Part model, mm, in its own coordinate system. A direction names the side the tool comes from. Coordinates: 2 decimals unless noted, no trailing zeros. Loops run counter-clockwise (first coordinate to the right, second up) from the corner with the lowest first, then second, coordinate; pieces in that order, holes last. Notation, with made-up numbers: (43, -4) - (53, -4) arc R38 cw to (53, 35) - close; hole circle Ø7 at (14.5, 87.5). An arc over 180 degrees is marked (long way). Use a Markdown table: item, result. Add a question column.
1. Band-saw the part on A-A, the plane z = 0.6. Give the cut face in (x, y) (3 decimals).
2. Wall check: probe 1 along X at (y, z) = (-5, 2.9); probe 2 along Y at (x, z) = (2.5, 0.95) (3 decimals); probe 3 along Y at (x, z) = (12.5, 0.55) (3 decimals). Give the ranges that are in metal, low to high. Write a range as [from, to].
3. Band-saw the part on B-B, the plane x = 9.5. Give the cut face in (y, z) (3 decimals), plus the area to 3 significant figures.
4. Pull direction X, two halves, no side cores. Call faces 3 (the flat face through (-19.05, 0, 2)), 4 (the flat face through (0, 0, 0)), 5 (the flat face through (0, -11.049, 2)): pulls with the +X half, pulls with the -X half, needs draft (parallel to the pull), parting line crosses it, or undercut.
5. Drop flat-ended pins along their axis: pin 1 (3 mm diameter, centred on x = 7, y = -1, fed in from +Z); pin 2 (10 mm diameter, centred on x = 15, y = 1, fed in from +Z). Give the stop position or say it passes through.
6. Band-saw the part on C-C, the plane y = 9. Give the cut face in (x, z), plus the area to 3 significant figures.
7. Band-saw the part on D-D, the plane x = -0.5. Give the cut face in (y, z) (3 decimals), plus the area to 3 significant figures.
8. 3-axis set-ups, long thin cutter, end or side, ignore diameter. For faces 1 (the flat face through (-0.267, -11.58, 3.025)), 2 (the flat face through (9.374, 5.089, 1.878)): which of +Z, -Z, +X, -X, +Y, -Y reach the whole face in a straight line?
from build123d import *

# Parameters (mm, degrees)
F0_W        = 38.1
F0_H        = 24.13
F1_DEPTH    = 3.81
F2_T1_DEPTH = 44.6320747894


# Not quite as in the source:
# - a fillet or chamfer that OpenCascade refuses, or shapes differently, is made with other operations: its cross-section is extruded or revolved along the edge and cut away or added


with BuildPart() as f1:
    # F0 (on Top) → F1 (new body)
    with BuildSketch(Plane.XY):
        Rectangle(F0_W, F0_H)
        Polygon((-0.029270627, -0.5935558801), (17.272, -11.049), (-17.330541254, -11.049), align=None, mode=Mode.SUBTRACT)
        Polygon((-18.034, -10.287), (-18.034, 10.287), (-1.0114642857, 0), align=None, mode=Mode.SUBTRACT)
        Polygon((-17.330541254, 11.049), (17.272, 11.049), (-0.029270627, 0.5935558801), align=None, mode=Mode.SUBTRACT)
        Polygon((0.9529230317, 0), (18.034, 10.3223774485), (18.034, -10.3223774485), align=None, mode=Mode.SUBTRACT)
    extrude(amount=F1_DEPTH)

    # F2: chamfer of 1.27 on 2 edges, made by hand

    # F2_s2 → F2_t1 (cut)
    with BuildSketch(Plane.YZ.offset(-22.3160373947)):
        Polygon((-12.065, 2.54), (-10.795, 3.81), (-12.065, 3.81), align=None)
        Polygon((12.065, 2.54), (10.795, 3.81), (12.065, 3.81), align=None)
    extrude(amount=F2_T1_DEPTH, mode=Mode.SUBTRACT)


solid = f1.part
Geometry check:
| question | item | result |
|---|---|---|
| 1 | outline | (-19.05, -12.065) - (19.05, -12.065) - (19.05, 12.065) - (-19.05, 12.065) - close; hole (-18.034, -10.287) - (-1.011, 0) - (-18.034, 10.287) - close; hole (-17.331, -11.049) - (17.272, -11.049) - (-0.029, -0.594) - close; hole (-17.331, 11.049) - (-0.029, 0.594) - (17.272, 11.049) - close; hole (0.953, 0) - (18.034, -10.322) - (18.034, 10.322) - close |
| 2 | probe 1 | x = [-19.05, -18.03], [-9.29, -7.32], [7.26, 9.23], [18.03, 19.05] |
| 2 | probe 2 | y = [-12.065, -11.049], [-2.122, -0.935], [0.935, 2.122], [11.049, 12.065] |
| 2 | probe 3 | y = [-12.065, -11.049], [-8.165, -6.978], [6.978, 8.165], [11.049, 12.065] |
| 3 | outline | (-12.065, 0) - (-11.049, 0) - (-11.049, 3.556) - (-12.065, 2.54) - close; (-6.352, 0) - (-5.165, 0) - (-5.165, 3.81) - (-6.352, 3.81) - close; (5.165, 0) - (6.352, 0) - (6.352, 3.81) - (5.165, 3.81) - close; (11.049, 0) - (12.065, 0) - (12.065, 2.54) - (11.049, 3.556) - close |
| 3 | area | 15.2 mm^2 |
| 4 | face 3 | pulls with the -X half |
| 4 | face 4 | needs draft |
| 4 | face 5 | undercut |
| 5 | pin 1 | passes through |
| 5 | pin 2 | stops at z = 3.81 |
| 6 | outline | (-19.05, 0) - (-18.03, 0) - (-18.03, 3.81) - (-19.05, 3.81) - close; (-15.9, 0) - (-13.94, 0) - (-13.94, 3.81) - (-15.9, 3.81) - close; (13.88, 0) - (15.85, 0) - (15.85, 3.81) - (13.88, 3.81) - close; (18.03, 0) - (19.05, 0) - (19.05, 3.81) - (18.03, 3.81) - close |
| 6 | area | 22.7 mm^2 |
| 7 | outline | (-12.065, 0) - (-11.049, 0) - (-11.049, 3.556) - (-12.065, 2.54) - close; (-0.878, 0) - (0.878, 0) - (0.878, 3.81) - (-0.878, 3.81) - close; (11.049, 0) - (12.065, 0) - (12.065, 2.54) - (11.049, 3.556) - close |
| 7 | area | 12.9 mm^2 |
| 8 | face 1 | +Z, +X, -X, -Y |
| 8 | face 2 | +Z, -Z |
